```python
from build123d import *
from OCP.BRepFilletAPI import BRepFilletAPI_MakeChamfer

# Parameters (mm, degrees)
SKETCH1_W           = 86
SKETCH1_H           = 86
BOSS_EXTRUDE1_DEPTH = 3
SKETCH2_W           = 79.8
SKETCH2_H           = 79.8
BOSS_EXTRUDE2_DEPTH = 4
SKETCH3_R           = 4
BOSS_EXTRUDE3_DEPTH = 9
SKETCH5_3_R         = 4
BOSS_EXTRUDE4_DEPTH = 6
FILLET1_R           = 1
CUT_EXTRUDE1_DEPTH  = 2.4
SKETCH5_R           = 1.6
CUT_EXTRUDE2_DEPTH  = 3.6
CUT_EXTRUDE3_DEPTH  = 2.5
SKETCH7_R           = 1.6
CUT_EXTRUDE4_DEPTH  = 6
SKETCH8_R           = 2.5
BOSS_EXTRUDE5_DEPTH = 9
CHAMFER1_SIZE       = 1
CHAMFER1_SIZE2      = 0.700207538


with BuildPart() as part:
    # Sketch1 → Boss-Extrude1 (new body)
    with BuildSketch(Plane.XY):
        Rectangle(SKETCH1_W, SKETCH1_H)
    extrude(amount=BOSS_EXTRUDE1_DEPTH)

    # Sketch2 → Boss-Extrude2 (add)
    with BuildSketch(Plane.XY.offset(3)):
        Rectangle(SKETCH2_W, SKETCH2_H)
    extrude(amount=BOSS_EXTRUDE2_DEPTH)

    # Sketch3 → Boss-Extrude3 (add)
    with BuildSketch(Plane.XY.offset(7)):
        with Locations((-34.14, 18.82)):
            Circle(SKETCH3_R)
        with Locations((-34.14, -9.12)):
            Circle(SKETCH3_R)
    extrude(amount=BOSS_EXTRUDE3_DEPTH)

    # Sketch5<3> → Boss-Extrude4 (add)
    with BuildSketch(Plane.XY.offset(7)):
        with Locations((17.93, 23.9)):
            Circle(SKETCH5_3_R)
        with Locations((16.66, -24.36)):
            Circle(SKETCH5_3_R)
    extrude(amount=BOSS_EXTRUDE4_DEPTH)

    # Fillet1
    fillet1_edges = [part.edges().sort_by_distance(p)[0] for p in [
        (-39.9, -39.9, 5),
        (39.9, -39.9, 5),
        (39.9, 39.9, 5),
        (-39.9, 39.9, 5),
        (-38.14, 18.82, 7),
        (-38.14, -9.12, 7),
        (13.93, 23.9, 7),
        (12.66, -24.36, 7),
    ]]
    fillet(fillet1_edges, radius=FILLET1_R)

    # Sketch4 → Cut-Extrude1 (cut)
    with BuildSketch(Plane.XY.offset(13)):
        Polygon((13.397970979, -24.36), (15.02898549, -27.185), (18.29101451, -27.185), (19.922029021, -24.36), (18.29101451, -21.535), (15.02898549, -21.535), align=None)
        Polygon((14.667970979, 23.9), (16.29898549, 21.075), (19.56101451, 21.075), (21.192029021, 23.9), (19.56101451, 26.725), (16.29898549, 26.725), align=None)
    extrude(amount=-CUT_EXTRUDE1_DEPTH, mode=Mode.SUBTRACT)

    # Sketch5 → Cut-Extrude2 (cut)
    with BuildSketch(Plane.XY.offset(10.6)):
        with Locations((17.93, 23.9)):
            Circle(SKETCH5_R)
        with Locations((16.66, -24.36)):
            Circle(SKETCH5_R)
    extrude(amount=-CUT_EXTRUDE2_DEPTH, mode=Mode.SUBTRACT)

    # Sketch6 → Cut-Extrude3 (cut)
    with BuildSketch(Plane.XY.offset(16)):
        Polygon((-37.402029021, 18.82), (-35.77101451, 15.995), (-32.50898549, 15.995), (-30.877970979, 18.82), (-32.50898549, 21.645), (-35.77101451, 21.645), align=None)
        Polygon((-37.402029021, -9.12), (-35.77101451, -11.945), (-32.50898549, -11.945), (-30.877970979, -9.12), (-32.50898549, -6.295), (-35.77101451, -6.295), align=None)
    extrude(amount=-CUT_EXTRUDE3_DEPTH, mode=Mode.SUBTRACT)

    # Sketch7 → Cut-Extrude4 (cut)
    with BuildSketch(Plane.XY.offset(13.5)):
        with Locations((-34.14, 18.82)):
            Circle(SKETCH7_R)
        with Locations((-34.14, -9.12)):
            Circle(SKETCH7_R)
    extrude(amount=-CUT_EXTRUDE4_DEPTH, mode=Mode.SUBTRACT)

    # Sketch8 → Boss-Extrude5 (add)
    with BuildSketch(Plane.XY.offset(7)):
        with Locations((25, 7)):
            Circle(SKETCH8_R)
    extrude(amount=BOSS_EXTRUDE5_DEPTH)

    # Chamfer1: one chamfer whose edges measure the first distance from different faces: ONE call of the kernel's chamfer builder (chamfer() names one face for all edges)
    chamfer1_edges_1 = [part.edges().sort_by_distance(p)[0] for p in [
        (0, -39.9, 7),
    ]]
    chamfer1_side_1 = [part.faces().sort_by_distance(p)[0] for p in [
        (0, -39.9, 5),
    ]]
    chamfer1_edges_2 = [part.edges().sort_by_distance(p)[0] for p in [
        (39.9, 0, 7),
    ]]
    chamfer1_side_2 = [part.faces().sort_by_distance(p)[0] for p in [
        (39.9, 0, 5),
    ]]
    chamfer1_edges_3 = [part.edges().sort_by_distance(p)[0] for p in [
        (0, 39.9, 7),
    ]]
    chamfer1_side_3 = [part.faces().sort_by_distance(p)[0] for p in [
        (0, 39.9, 5),
    ]]
    chamfer1_edges_4 = [part.edges().sort_by_distance(p)[0] for p in [
        (-39.9, 0, 7),
    ]]
    chamfer1_side_4 = [part.faces().sort_by_distance(p)[0] for p in [
        (-39.9, 0, 5),
    ]]
    chamfer1_edges_5 = [part.edges().sort_by_distance(p)[0] for p in [
        (-39.607106781, 39.607106781, 7),
    ]]
    chamfer1_side_5 = [part.faces().sort_by_distance(p)[0] for p in [
        (-39.607106781, 39.607106781, 5),
    ]]
    chamfer1_edges_6 = [part.edges().sort_by_distance(p)[0] for p in [
        (-39.607106781, -39.607106781, 7),
    ]]
    chamfer1_side_6 = [part.faces().sort_by_distance(p)[0] for p in [
        (-39.607106781, -39.607106781, 5),
    ]]
    chamfer1_edges_7 = [part.edges().sort_by_distance(p)[0] for p in [
        (39.607106781, -39.607106781, 7),
    ]]
    chamfer1_side_7 = [part.faces().sort_by_distance(p)[0] for p in [
        (39.607106781, -39.607106781, 5),
    ]]
    chamfer1_edges_8 = [part.edges().sort_by_distance(p)[0] for p in [
        (39.607106781, 39.607106781, 7),
    ]]
    chamfer1_side_8 = [part.faces().sort_by_distance(p)[0] for p in [
        (39.607106781, 39.607106781, 5),
    ]]
    chamfer1 = BRepFilletAPI_MakeChamfer(part.part.solid().wrapped)
    for e in chamfer1_edges_1:
        chamfer1.Add(CHAMFER1_SIZE, CHAMFER1_SIZE2, e.wrapped, chamfer1_side_1[0].wrapped)  # the first distance lies on this face
    for e in chamfer1_edges_2:
        chamfer1.Add(CHAMFER1_SIZE, CHAMFER1_SIZE2, e.wrapped, chamfer1_side_2[0].wrapped)  # the first distance lies on this face
    for e in chamfer1_edges_3:
        chamfer1.Add(CHAMFER1_SIZE, CHAMFER1_SIZE2, e.wrapped, chamfer1_side_3[0].wrapped)  # the first distance lies on this face
    for e in chamfer1_edges_4:
        chamfer1.Add(CHAMFER1_SIZE, CHAMFER1_SIZE2, e.wrapped, chamfer1_side_4[0].wrapped)  # the first distance lies on this face
    for e in chamfer1_edges_5:
        chamfer1.Add(CHAMFER1_SIZE, CHAMFER1_SIZE2, e.wrapped, chamfer1_side_5[0].wrapped)  # the first distance lies on this face
    for e in chamfer1_edges_6:
        chamfer1.Add(CHAMFER1_SIZE, CHAMFER1_SIZE2, e.wrapped, chamfer1_side_6[0].wrapped)  # the first distance lies on this face
    for e in chamfer1_edges_7:
        chamfer1.Add(CHAMFER1_SIZE, CHAMFER1_SIZE2, e.wrapped, chamfer1_side_7[0].wrapped)  # the first distance lies on this face
    for e in chamfer1_edges_8:
        chamfer1.Add(CHAMFER1_SIZE, CHAMFER1_SIZE2, e.wrapped, chamfer1_side_8[0].wrapped)  # the first distance lies on this face
    add(Compound.cast(chamfer1.Shape()), mode=Mode.REPLACE)


solid = part.part
```
For this review, take the finished solid that the model builds, in its own axes (mm). A direction names the side the tool comes from. Round coordinates to 2 decimals unless told otherwise and drop trailing zeros. Order: outer loops, then holes, each group sorted by start corner. A loop starts at its lowest first (then second) coordinate and runs counter-clockwise, first axis right, second up.
Q1. Wall thickness on line 1 (Y direction, x = -34.14, z = 8.8); line 2 (Z direction, x = 15.5, y = -31); line 3 (X direction, y = 19, z = 11.25): over which ranges is each line inside the solid? List them lowest first.
Findings below:
line 1: y = -13.12 to -10.72, -7.52 to -5.12, 14.82 to 17.22, 20.42 to 22.82
line 2: z = 0 to 7
line 3: x = -38.14 to -35.73, -32.55 to -30.14
Q2. We need section B-B, the plane x = -14. Give the boundary of the cut face in (y, z), plus the area to 4 significant figures.
Findings below:
outline: (-43, 0) - (43, 0) - (43, 3) - (39.9, 3) - (39.9, 6) - (39.2, 7) - (-39.2, 7) - (-39.9, 6) - (-39.9, 3) - (-43, 3) - close
area: 576.5 mm2
Q3. We need section A-A, the plane z = 9.5. State how many separate pieces and enclosed holes the cut face has, plus the area to 3 significant figures.
Findings below:
separate pieces: 5
enclosed holes: 4
area: 189 mm2
Q4. We need section D-D, the plane x = 25. Give the boundary of the cut face in (y, z), plus the area to 4 significant figures.
Findings below:
outline: (-43, 0) - (43, 0) - (43, 3) - (39.9, 3) - (39.9, 6) - (39.2, 7) - (9.5, 7) - (9.5, 16) - (4.5, 16) - (4.5, 7) - (-39.2, 7) - (-39.9, 6) - (-39.9, 3) - (-43, 3) - close
area: 621.5 mm2
Q5. Mouldability with a two-part tool opening along Y and no side actions: class faces 4 (the flat face through (-37, 17, 16)), 5 (the flat face through (17, -24, 7)) as pulls with the +Y half, pulls with the -Y half, needs draft (parallel to the pull), parting line crosses it, or undercut.
Findings below:
face 4: needs draft
face 5: undercut
Q6. Machinability: for faces 1 (the flat face through (39.9, -1, 4)), 2 (the flat face through (-34.2, -12.1, 16)), 3 (the flat face through (-36.6, 17.43, 14.77)), which of the approach directions +Z, -Z, +X, -X, +Y, -Y give a long, thin tool a straight path to every point of the face, cutting with its end or side? Answer none if there is none.
Findings below:
face 1: +Z, +X, +Y, -Y
face 2: +Z, +X, -X, +Y, -Y
face 3: +Z
Q7. Insertion check: P1, Ø1.7, axis at x = 18.5, y = 23, coming from the +Z side; P2, Ø3.5, axis at x = -33.5, y = 19.5, coming from the +Z side; P3, Ø0.8, axis at x = -33.5, z = 14.5, coming from the +Y side. Each pin has a flat end and moves straight along its axis. Give the tip position at first contact, or say it passes through.
Findings below:
P1: stops at z = 10.6
P2: stops at z = 13.5
P3: stops at y = 22.81
